Source: three-view drawing plus pictorial views. Frame: mm from the lowest corner of the part. A direction names the side the tool comes from. Give positions to 0.01 mm unless a question says otherwise; leave off trailing zeros. Write each loop counter-clockwise with the first axis right and the second up, starting at its lowest first coordinate (ties: lowest second). Pieces come first, ordered by that corner, then holes.
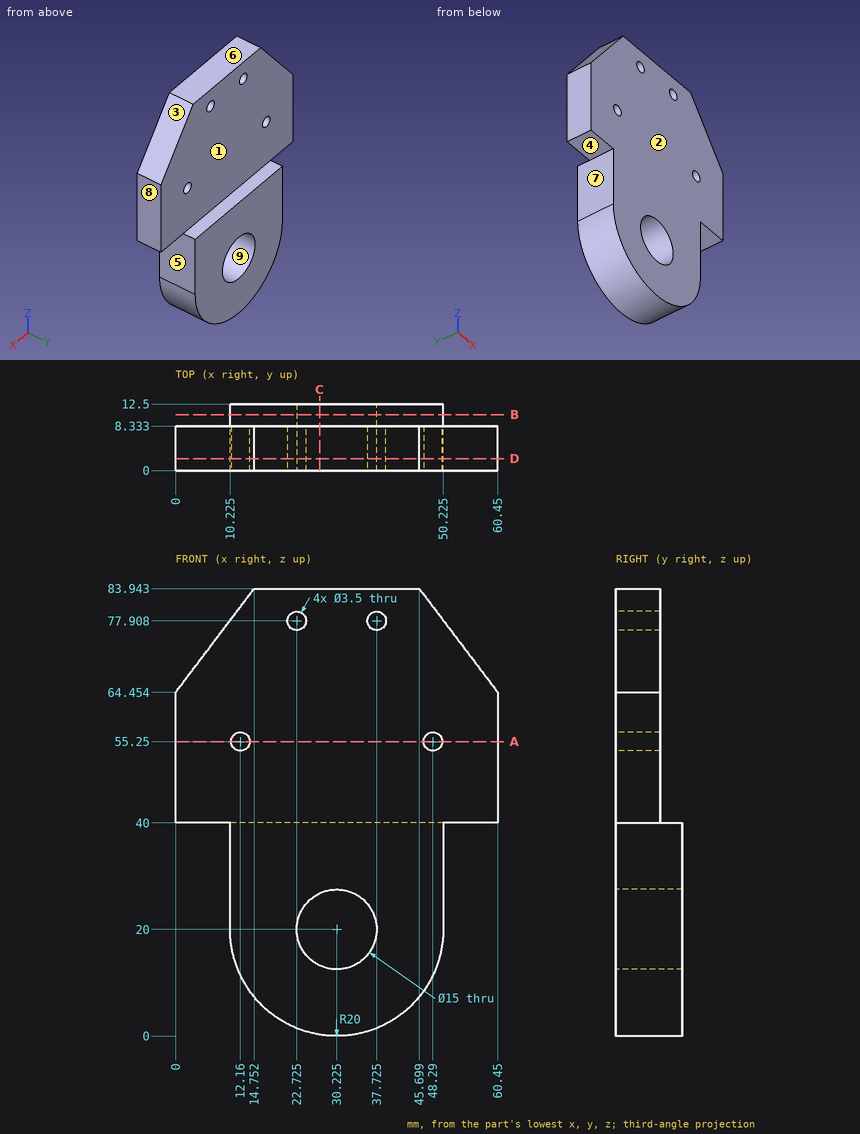
Q1. Pin query (flat end, axial travel): P1, Ø1.5, axis at y = 8, z = 55.5, coming from the -X side; P2, Ø4.5, axis at x = 37.73, z = 77.91, coming from the +Y side; P3, Ø4, axis at x = 3, y = 2.5, coming from the -Z side; P4, Ø4, axis at y = 8, z = 32, coming from the -X side (1 decimal). Return the tip coordinate at first contact, or that it passes through.
Filled sheet:
P1: stops at x = 0
P2: stops at y = 8.33
P3: stops at z = 40
P4: stops at x = 10.2
Q2. Section D-D on y = 2.25. Count the separate pieces of the cut face and the enclosed holes in it, plus the area to 3 significant figures.
Filled sheet:
separate pieces: 1
enclosed holes: 5
area: 3,580 mm2
Q3. Ray query, line 1 along X through (y, z) = (1.25, 77.5) (1 decimal); line 2 along Z through (x, y) = (35.5, 3.5) (1 decimal); line 3 along Y through (x, z) = (29.5, 54). Return the intervals inside material, ascending.
Filled sheet:
line 1: x = 9.9 to 21, 24.4 to 36, 39.4 to 50.6
line 2: z = 0.7 to 14.7, 25.3 to 83.9
line 3: y = 0 to 8.33
Q4. Pull-direction query (X, two-part tool) for the marked faces 6, 7, 8 and 9; classes: released by +X, released by -X, zero draft, split by the parting line, or undercut.
Filled sheet:
face 6: zero draft
face 7: released by -X
face 8: released by +X
face 9: undercut
Q5. Access query for the marked faces 1, 2, 3, 4 and 5. Directions: +Z, -Z, +X, -X, +Y, -Y. A direction counts if a zero-diameter tool reaches every point of the face in a straight line with its end or side. Return the directions, or none.
Filled sheet:
face 1: +Z, +X, -X, +Y
face 2: +Z, -Z, +X, -X, -Y
face 3: +Z, +X, +Y, -Y
face 4: -Z, -X, +Y, -Y
face 5: -Z, +X, +Y, -Y
Q6. Section C-C on x = 27. Output: boundary loops of the cut face in (y, z).
Filled sheet:
outline: (0, 0.26) - (12.5, 0.26) - (12.5, 13.23) - (0, 13.23) - close; (0, 26.77) - (12.5, 26.77) - (12.5, 40) - (8.33, 40) - (8.33, 83.94) - (0, 83.94) - close
Q7. Section B-B on y = 10.5. Output: boundary loops of the cut face in (x, z) (1 decimal), plus the area to 3 significant figures.
Filled sheet:
outline: (10.2, 20) arc R20 ccw to (50.2, 20) - (50.2, 40) - (10.2, 40) - close; hole circle Ø15 at (30.2, 20)
area: 1,250 mm2
Q8. Section A-A on z = 55.25. Output: boundary loops of the cut face in (x, y).
Filled sheet:
outline: (0, 0) - (10.41, 0) - (10.41, 8.33) - (0, 8.33) - close; (13.91, 0) - (46.54, 0) - (46.54, 8.33) - (13.91, 8.33) - close; (50.04, 0) - (60.45, 0) - (60.45, 8.33) - (50.04, 8.33) - close
